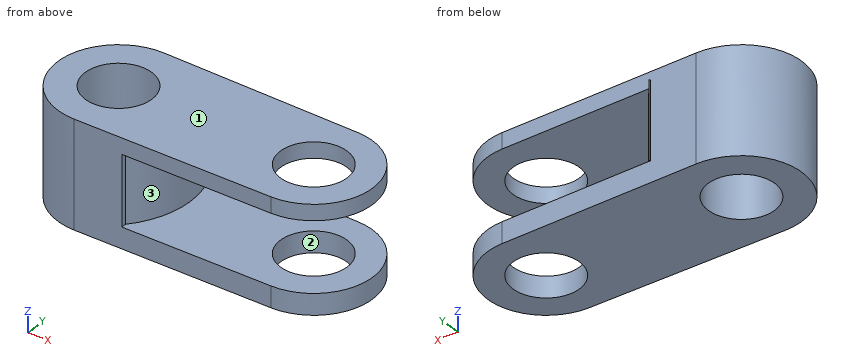
```python
from build123d import *

# Parameters (mm, degrees)
F0_R     = 15.9206607186
F1_DEPTH = 50.8
F2_DEPTH = 50.8
F3_W     = 100.2022400498
F3_H     = 33.2709047943
F4_DEPTH = 77.724
F7_DEPTH = 36.83


with BuildPart() as f1:
    # F0 (on Top) → F1 (new body)
    with BuildSketch(Plane.XY):
        with BuildLine():
            ThreePointArc((-46.3083671537, -28.9735284728), (-17.6046094791, 0), (-46.3083671537, 28.9735284728))
            ThreePointArc((-46.3083671537, 28.9735284728), (-75.5542018517, 0), (-46.3083671537, -28.9735284728))
        make_face()
        with Locations((-46.5794056654, 0)):
            Circle(F0_R, mode=Mode.SUBTRACT)
    extrude(amount=F1_DEPTH)

    # F0 (on Top) → F2 (join)
    with BuildSketch(Plane.XY):
        with BuildLine():
            Line((46.8422925338, 28.1021324953), (-46.3083671537, 28.9735284728))
            ThreePointArc((-46.3083671537, 28.9735284728), (-17.6046094791, 0), (-46.3083671537, -28.9735284728))
            Line((-46.3083671537, -28.9735284728), (46.8422925338, -28.1021324953))
            ThreePointArc((46.8422925338, -28.1021324953), (74.682767747, 0), (46.8422925338, 28.1021324953))
        make_face()
        with Locations((46.5794056654, 0)):
            Circle(F0_R, mode=Mode.SUBTRACT)
    extrude(amount=F2_DEPTH)

    # F3 (on face) → F4 (cut)
    with BuildSketch(Plane(origin=(0.26696269, -28.537830484, 0), x_dir=(0.9999562477, 0.0093542854, 0), z_dir=(0.0093542854, -0.9999562477, 0))):
        with Locations((26.0913781822, 26.6495971009)):
            Rectangle(F3_W, F3_H)
    extrude(amount=-F4_DEPTH, mode=Mode.SUBTRACT)

    # F6 (on face) → F7 (join)
    with BuildSketch(Plane.XY.offset(10.0141447037)):
        with BuildLine():
            Line((-24.3764873594, 29.5255221426), (-24.3764873594, -27.0263291895))
            ThreePointArc((-24.3764873594, -27.0263291895), (-13.2836024282, 1.2495964766), (-24.3764873594, 29.5255221426))
        make_face()
    extrude(amount=F7_DEPTH)


solid = f1.part
```
Geometry: final body of the model. Coordinates: model frame, mm. Face numbers are marked on the shaded views. Give positions to 0.01 mm unless a question says otherwise; leave off trailing zeros. Loops run counter-clockwise (first coordinate to the right, second up) from the corner with the lowest first, then second, coordinate; pieces in that order, holes last. Notation, with made-up numbers: (71.5, -36.5) -> (108.5, -36.5) arc R19 cw to (108.5, -27.5) -> close; hole circle Ø10 at (46, 17). An arc over 180 degrees is marked (long way). Return JSON: item names as keys, results as strings.
Item 1: Pin query (flat end, axial travel): P1, Ø1, axis at y = -20, z = 45.5, coming from the -X side; P2, Ø2, axis at x = -25.5, z = 35, coming from the +Y side; P3, Ø1, axis at x = 32, y = -3.5, coming from the +Z side; P4, Ø12, axis at x = -14, z = 10, coming from the -Y side. Return the tip coordinate at first contact, or that it passes through.
Filled in:
{"P1": "x = -68.01", "P2": "y = 28.79", "P3": "through", "P4": "y = -28.73"}
Item 2: Section D-D, the plane y = 9. Output: boundary loops of the cut face in (x, z).
Filled in:
{"outline": "(-74.12, 0) -> (-59.71, 0) -> (-59.71, 50.8) -> (-74.12, 50.8) -> close; (-33.45, 0) -> (33.45, 0) -> (33.45, 10.01) -> (-14.01, 10.01) -> (-14.01, 43.29) -> (33.45, 43.29) -> (33.45, 50.8) -> (-33.45, 50.8) -> close; (59.71, 0) -> (73.2, 0) -> (73.2, 10.01) -> (59.71, 10.01) -> close; (59.71, 43.29) -> (73.2, 43.29) -> (73.2, 50.8) -> (59.71, 50.8) -> close"}
Item 3: Mould query, pull axis Y, two halves, no side actions, for the marked faces 1, 2 and 3. Classes: released by +Y, released by -Y, zero draft, split by the parting line, or undercut.
Filled in:
{"face 1": "zero draft", "face 2": "undercut", "face 3": "split by the parting line"}
Item 4: Line query: line 1 (X direction, y = 1, z = 23.5); line 2 (Z direction, x = 31, y = -20.5); line 3 (X direction, y = -4.5, z = 7.5). Output: solid intervals per line, ascending.
Filled in:
{"line 1": "-75.54 to -62.47, -30.69 to -13.28", "line 2": "0 to 10.01, 43.29 to 50.8", "line 3": "-75.2 to -61.85, -31.31 to 31.31, 61.85 to 74.32"}
Item 5: Section B-B, the plane y = -9.5. Output: boundary loops of the cut face in (x, z), plus the area to 3 significant figures.
Filled in:
{"outline": "(-73.95, 0) -> (-59.36, 0) -> (-59.36, 50.8) -> (-73.95, 50.8) -> close; (-33.8, 0) -> (33.8, 0) -> (33.8, 10.01) -> (-14.7, 10.01) -> (-14.7, 43.29) -> (33.8, 43.29) -> (33.8, 50.8) -> (-33.8, 50.8) -> close; (59.36, 0) -> (73.03, 0) -> (73.03, 10.01) -> (59.36, 10.01) -> close; (59.36, 43.29) -> (73.03, 43.29) -> (73.03, 50.8) -> (59.36, 50.8) -> close", "area": "2,800 mm^2"}
Item 6: Section C-C, the plane x = 22. Output: boundary loops of the cut face in (y, z).
Filled in:
{"outline": "(-28.33, 0) -> (28.33, 0) -> (28.33, 10.01) -> (-28.33, 10.01) -> close; (-28.33, 43.29) -> (28.33, 43.29) -> (28.33, 50.8) -> (-28.33, 50.8) -> close"}
